```python
from build123d import *

# Parameters (mm, degrees)
SKETCH1_R                        = 82.55
EXTRUDE1_DEPTH                   = 19.05
F_1_1_DIAMETER_HOLE2_D           = 25.4
F_1_1_DIAMETER_HOLE2_DEPTH       = 19.05
F_1_2_20_TAPPED_HOLE1_AT_2_COUNT = 2
F_1_2_20_TAPPED_HOLE1_AT_2_PITCH = 120.983748909
F_1_2_20_TAPPED_HOLE1_AT_3_COUNT = 2
F_1_2_20_TAPPED_HOLE1_AT_3_PITCH = 120.983748909
F_1_2_CLEARANCE_HOLE1_AT_2_COUNT = 2
F_1_2_CLEARANCE_HOLE1_AT_2_PITCH = 120.983748909
F_1_2_CLEARANCE_HOLE1_AT_3_COUNT = 2
F_1_2_CLEARANCE_HOLE1_AT_3_PITCH = 120.983748909
CHAMFER6_SIZE                    = 1.524


with BuildPart() as part:
    # Sketch1 → Extrude1 (new body)
    with BuildSketch(Plane(origin=(0, 0, 0), x_dir=(1, 0, 0), z_dir=(0, 1, 0))):
        with Locations(Location((0, 0, 0), (0, 0, 270))):  # turned: the seam where the file's is
            Circle(SKETCH1_R)
    extrude(amount=EXTRUDE1_DEPTH)

    # 1 _1_ Diameter Hole2
    with Locations(Plane(origin=(0, 19.05, 0), x_dir=(-1, 0, 0), z_dir=(0, 1, 0))):
        with Locations((0, 0)):
            Hole(F_1_1_DIAMETER_HOLE2_D / 2, depth=F_1_1_DIAMETER_HOLE2_DEPTH)

    # Sketch12 → 1_2-20 Tapped Hole1 (revolve, cut)
    with BuildSketch(Plane(origin=(0, 19.05, 69.85), x_dir=(0, 0, 1), z_dir=(1, 0, 0))):
        Polygon((0, 0), (0, 19.05), (6.985, 19.05), (6.35, 18.319516061), (6.35, 0.730483939), (6.985, 0), align=None)
    f_1_2_20_tapped_hole1 = revolve(axis=Axis((0, 25.4, 69.85), (0, -1, 0)), mode=Mode.SUBTRACT)

    # 1_2-20 Tapped Hole1 at 2: 1_2-20 Tapped Hole1 ×2
    with Locations(*[Vector(-0.5, 0, -0.866025404) * (i * F_1_2_20_TAPPED_HOLE1_AT_2_PITCH) for i in range(1, F_1_2_20_TAPPED_HOLE1_AT_2_COUNT)]):
        add(f_1_2_20_tapped_hole1, mode=Mode.SUBTRACT)

    # 1_2-20 Tapped Hole1 at 3: 1_2-20 Tapped Hole1 ×2
    with Locations(*[Vector(0.5, 0, -0.866025404) * (i * F_1_2_20_TAPPED_HOLE1_AT_3_PITCH) for i in range(1, F_1_2_20_TAPPED_HOLE1_AT_3_COUNT)]):
        add(f_1_2_20_tapped_hole1, mode=Mode.SUBTRACT)

    # Sketch14 → 1_2 Clearance Hole1 (revolve, cut)
    with BuildSketch(Plane(origin=(0, 19.05, -69.85), x_dir=(0, 0, 1), z_dir=(1, 0, 0))):
        Polygon((0, 0), (0, 19.05), (7.62, 19.05), (6.94563, 18.274226057), (6.94563, 0.775773943), (7.62, 0), align=None)
    f_1_2_clearance_hole1 = revolve(axis=Axis((0, 25.4, -69.85), (0, -1, 0)), mode=Mode.SUBTRACT)

    # 1_2 Clearance Hole1 at 2: 1_2 Clearance Hole1 ×2
    with Locations(*[Vector(-0.5, 0, 0.866025404) * (i * F_1_2_CLEARANCE_HOLE1_AT_2_PITCH) for i in range(1, F_1_2_CLEARANCE_HOLE1_AT_2_COUNT)]):
        add(f_1_2_clearance_hole1, mode=Mode.SUBTRACT)

    # 1_2 Clearance Hole1 at 3: 1_2 Clearance Hole1 ×2
    with Locations(*[Vector(0.5, 0, 0.866025404) * (i * F_1_2_CLEARANCE_HOLE1_AT_3_PITCH) for i in range(1, F_1_2_CLEARANCE_HOLE1_AT_3_COUNT)]):
        add(f_1_2_clearance_hole1, mode=Mode.SUBTRACT)

    # Chamfer6
    chamfer6_edges = [part.edges().sort_by_distance(p)[0] for p in [
        (0, 0, -82.55),
        (0, 19.05, -82.55),
    ]]
    chamfer(chamfer6_edges, length=CHAMFER6_SIZE)


solid = part.part
```
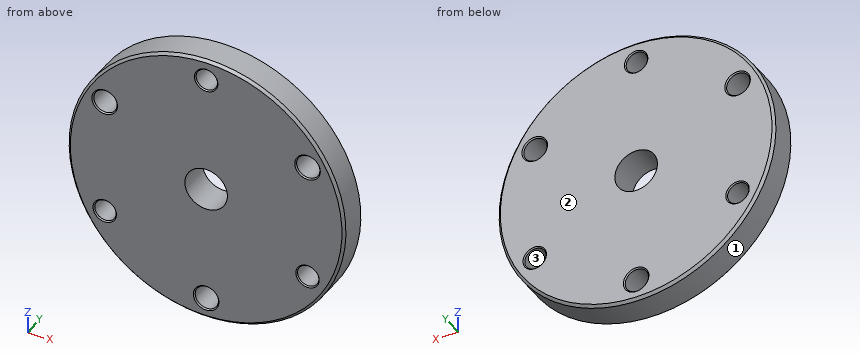
Can you work these out from the model? Positions are in its coordinate system, mm. Face numbers are marked on the shaded views. Round coordinates to 2 decimals unless told otherwise and drop trailing zeros. Order: outer loops, then holes, each group sorted by start corner. A loop starts at its lowest first (then second) coordinate and runs counter-clockwise, first axis right, second up.
(1) If we section it at A-A (x = 0): Please give me the cut outline in (y, z) (3 decimals).
Results are:
outline: (0, -81.026) - (1.524, -82.55) - (17.526, -82.55) - (19.05, -81.026) - (19.05, -77.47) - (18.274, -76.796) - (0.776, -76.796) - (0, -77.47) - close; (0, -62.23) - (0.776, -62.904) - (18.274, -62.904) - (19.05, -62.23) - (19.05, -12.7) - (0, -12.7) - close; (0, 12.7) - (19.05, 12.7) - (19.05, 62.865) - (18.32, 63.5) - (0.73, 63.5) - (0, 62.865) - close; (0, 76.835) - (0.73, 76.2) - (18.32, 76.2) - (19.05, 76.835) - (19.05, 81.026) - (17.526, 82.55) - (1.524, 82.55) - (0, 81.026) - close
(2) If we section it at B-B (z = 0): Please give me the cut outline in (x, y).
Results are:
outline: (-82.55, 1.52) - (-81.03, 0) - (-12.7, 0) - (-12.7, 19.05) - (-81.03, 19.05) - (-82.55, 17.53) - close; (12.7, 0) - (81.03, 0) - (82.55, 1.52) - (82.55, 17.53) - (81.03, 19.05) - (12.7, 19.05) - close
(3) If I drill on L1, parallel to X at y = 5.25, z = -39.5; L2, parallel to X at y = 9.25, z = -35; L3, parallel to Z at x = -1, y = 2, over which ranges is the centre line in solid material (lowest first)?
Results are:
L1: x = -72.49 to -64.9, -56.09 to 56.09, 64.9 to 72.49
L2: x = -74.76 to -66.84, -54.14 to 54.14, 66.84 to 74.76
L3: z = -82.54 to -76.72, -62.98 to -12.66, 12.66 to 63.58, 76.12 to 82.54
(4) I'm going to push flat-ended pins straight in: pin 1 (11.5 mm diameter, centred on x = 60.49, z = -34.93, fed in from +Y); pin 2 (6 mm diameter, centred on x = -14, y = 7, fed in from -Z); pin 3 (8 mm diameter, centred on x = 16, y = 9, fed in from +Z); pin 4 (6 mm diameter, centred on x = 25, y = 12.5, fed in from -Z). Where does each tip first touch, or does it pass through?
Results are:
pin 1: passes through
pin 2: stops at z = -81.81
pin 3: stops at z = 81.67
pin 4: stops at z = -79.56
(5) If we section it at C-C (y = 13): Please give me the cut outline in (x, z) (3 decimals).
Results are:
outline: circle Ø165.1 at (0, 0); hole circle Ø13.891 at (-60.492, 34.925); hole circle Ø12.7 at (-60.492, -34.925); hole circle Ø25.4 at (0, 0); hole circle Ø13.891 at (0, -69.85); hole circle Ø12.7 at (0, 69.85); hole circle Ø13.891 at (60.492, 34.925); hole circle Ø12.7 at (60.492, -34.925)
(6) If we section it at D-D (z = -34): Count the separate pieces of the cut face and the enclosed holes in it, plus the area to 3 significant figures.
Results are:
separate pieces: 3
enclosed holes: 0
area: 2,380 mm2
(7) We'd pull the mould along X, two halves only. Please class the marked faces 1, 2 and 3: +X half, -X half, draft (parallel to the pull), parting line (faces both ways), or undercut.
Results are:
face 1: parting line
face 2: draft
face 3: undercut
